The listing builds one solid part. Answer for the finished solid, in the listing's coordinates (mm). A direction names the side the tool comes from. Give positions to 0.01 mm unless a question says otherwise; leave off trailing zeros. Write each loop counter-clockwise with the first axis right and the second up, starting at its lowest first coordinate (ties: lowest second). Pieces come first, ordered by that corner, then holes.
```python
from build123d import *

# Parameters (mm, degrees)
SKETCH1_W           = 49.5
SKETCH1_H           = 61.5
BOSS_EXTRUDE1_DEPTH = 23.75
SKETCH2_W           = 46
SKETCH2_H           = 58
CUT_EXTRUDE1_DEPTH  = 22
SKETCH3_W           = 3
SKETCH3_H           = 16
CUT_EXTRUDE2_DEPTH  = 1.75
SKETCH7_W           = 3
SKETCH7_H           = 5
BOSS_EXTRUDE2_DEPTH = 4
SKETCH11_W          = 37.5
SKETCH11_H          = 61.5
BOSS_EXTRUDE3_DEPTH = 15
SKETCH12_W          = 34
SKETCH12_H          = 57
CUT_EXTRUDE3_DEPTH  = 15


with BuildPart() as part:
    # Sketch1 → Boss-Extrude1 (new body)
    with BuildSketch(Plane(origin=(0, 0, 0), x_dir=(1, 0, 0), z_dir=(0, 1, 0))):
        with Locations((-113.412024913, -45.391200727)):
            Rectangle(SKETCH1_W, SKETCH1_H)
    extrude(amount=BOSS_EXTRUDE1_DEPTH)

    # Sketch2 → Cut-Extrude1 (cut)
    with BuildSketch(Plane(origin=(0, 0, 0), x_dir=(-1, 0, 0), z_dir=(0, -1, 0))):
        with Locations((113.412024913, -45.391200727)):
            Rectangle(SKETCH2_W, SKETCH2_H)
    extrude(amount=-CUT_EXTRUDE1_DEPTH, mode=Mode.SUBTRACT)

    # Sketch3 → Cut-Extrude2 (cut)
    with BuildSketch(Plane(origin=(0, 22, 0), x_dir=(-1, 0, 0), z_dir=(0, -1, 0))):
        with Locations((91.912024913, -66.391200727)):
            Rectangle(SKETCH3_W, SKETCH3_H)
        with Locations((91.912024913, -24.391200727)):
            Rectangle(SKETCH3_W, SKETCH3_H)
        with Locations((91.912024913, -45.391200727)):
            Rectangle(SKETCH3_W, SKETCH3_H)
    extrude(amount=-CUT_EXTRUDE2_DEPTH, mode=Mode.SUBTRACT)

    # Sketch7 → Boss-Extrude2 (add)
    with BuildSketch(Plane(origin=(0, 22, 0), x_dir=(-1, 0, 0), z_dir=(0, -1, 0))):
        with Locations((91.912024913, -55.891200727)):
            Rectangle(SKETCH7_W, SKETCH7_H)
        with Locations((91.912024913, -34.891200727)):
            Rectangle(SKETCH7_W, SKETCH7_H)
    extrude(amount=BOSS_EXTRUDE2_DEPTH)

    # Sketch11 → Boss-Extrude3 (add)
    with BuildSketch(Plane(origin=(0, 23.75, 0), x_dir=(1, 0, 0), z_dir=(0, 1, 0))):
        with Locations((-119.412024913, -45.391200727)):
            Rectangle(SKETCH11_W, SKETCH11_H)
    extrude(amount=BOSS_EXTRUDE3_DEPTH)

    # Sketch12 → Cut-Extrude3 (cut)
    with BuildSketch(Plane(origin=(0, 38.75, 0), x_dir=(1, 0, 0), z_dir=(0, 1, 0))):
        with Locations((-119.412024913, -45.391200727)):
            Rectangle(SKETCH12_W, SKETCH12_H)
    extrude(amount=-CUT_EXTRUDE3_DEPTH, mode=Mode.SUBTRACT)


solid = part.part
```
Item 1: A cutting plane is placed at A-A, the plane x = -91.5. Give the vertices of the cut face in (y, z).
Conclusion:
outline: (0, 14.64) - (23.75, 14.64) - (23.75, 16.39) - (0, 16.39) - close; (0, 74.39) - (23.75, 74.39) - (23.75, 76.14) - (0, 76.14) - close; (18, 32.39) - (23.75, 32.39) - (23.75, 37.39) - (18, 37.39) - close; (18, 53.39) - (23.75, 53.39) - (23.75, 58.39) - (18, 58.39) - close
Item 2: Consider probe 1 along X at (y, z) = (22.5, 71.5); probe 2 along Z at (x, y) = (-114, 7); probe 3 along X at (y, z) = (26, 61). Determine where each line is inside the solid, lowest interval first.
Conclusion:
probe 1: x = -138.16 to -93.41, -90.41 to -88.66
probe 2: z = 14.64 to 16.39, 74.39 to 76.14
probe 3: x = -138.16 to -136.41, -102.41 to -100.66
Item 3: A cutting plane is placed at D-D, the plane x = -133. Give the vertices of the cut face in (y, z).
Conclusion:
outline: (0, 14.64) - (38.75, 14.64) - (38.75, 16.89) - (23.75, 16.89) - (23.75, 73.89) - (38.75, 73.89) - (38.75, 76.14) - (0, 76.14) - (0, 74.39) - (22, 74.39) - (22, 16.39) - (0, 16.39) - close
Item 4: Which of the six approach directions +Z, -Z, +X, -X, +Y, -Y give full straight-line access (tool end or side, diameter ignored) to faces 1 (the face through (-96, 23.75, 45)), 2 (the face through (-102.412, 31, 46)), 3 (the face through (-113, 12, 74.391)), 4 (the face through (-93.412, 23, 25))?
Conclusion:
face 1: +Z, -Z, +X, +Y
face 2: +Y
face 3: -Y
face 4: +Y, -Y
Item 5: Each of these flat-tipped pins is pushed along its axis until it touches: P1, Ø4.5, axis at y = 30.5, z = 45.5, coming from the +X side; P2, Ø17, axis at x = -127, z = 37.5, coming from the +Y side; P3, Ø2, axis at x = -106.5, z = 52, coming from the -Y side. Where does it stop, or does it pass through?
Conclusion:
P1: stops at x = -100.66
P2: stops at y = 23.75
P3: stops at y = 22
Item 6: A cutting plane is placed at B-B, the plane z = 26.5. Give the vertices of the cut face in (x, y).
Conclusion:
outline: (-138.16, 0) - (-136.41, 0) - (-136.41, 22) - (-93.41, 22) - (-93.41, 23.75) - (-100.66, 23.75) - (-100.66, 38.75) - (-102.41, 38.75) - (-102.41, 23.75) - (-136.41, 23.75) - (-136.41, 38.75) - (-138.16, 38.75) - close; (-90.41, 0) - (-88.66, 0) - (-88.66, 23.75) - (-90.41, 23.75) - close
Item 7: Determine the mould class of faces 5 (the face through (-137, 0, 45)), 6 (the face through (-93.412, 20, 35)), 7 (the face through (-138.162, 19, 46)) for opening direction X: pulls with the +X half, pulls with the -X half, needs draft (parallel to the pull), parting line crosses it, or undercut.
Conclusion:
face 5: needs draft
face 6: undercut
face 7: pulls with the -X half
Item 8: A cutting plane is placed at C-C, the plane y = 5. Give the vertices of the cut face in (x, z), plus the area to 3 significant figures.
Conclusion:
outline: (-138.16, 14.64) - (-88.66, 14.64) - (-88.66, 76.14) - (-138.16, 76.14) - close; hole (-136.41, 16.39) - (-90.41, 16.39) - (-90.41, 74.39) - (-136.41, 74.39) - close
area: 376 mm2
